Read the model definition and answer for the solid it produces. Units are mm, in the model's axes. A direction names the side the tool comes from. Give positions to 0.01 mm unless a question says otherwise; leave off trailing zeros. Order: outer loops, then holes, each group sorted by start corner. A loop starts at its lowest first (then second) coordinate and runs counter-clockwise, first axis right, second up. Notation, with made-up numbers: (-25.75, 30.25) - (18.25, 30.25) arc R3 ccw to (18.25, 34.25) - close; hole circle Ø9 at (55, 23). An arc over 180 degrees is marked (long way). Write item = value, one per line.
```python
from build123d import *

# Parameters (mm, degrees)
F0_W     = 40
F0_H     = 20
F0_R     = 10
F1_DEPTH = 30
F2_DEPTH = 30


with BuildPart() as f1:
    # F0 (on Front) → F1 (new body)
    with BuildSketch(Plane.XZ):
        with BuildLine():
            ThreePointArc((-20.300006, -30.491507), (-17.371073, -37.562575), (-10.300006, -40.491507))
            Line((-10.300006, -40.491507), (89.699994, -40.491507))
            ThreePointArc((89.699994, -40.491507), (96.771062, -37.562575), (99.699994, -30.491507))
            ThreePointArc((99.699994, -30.491507), (102.628927, -23.420439), (109.699994, -20.491507))
            Line((109.699994, -20.491507), (119.699994, -20.491507))
            ThreePointArc((119.699994, -20.491507), (126.771062, -17.562575), (129.699994, -10.491507))
            Line((129.699994, -10.491507), (129.699994, 69.508493))
            ThreePointArc((129.699994, 69.508493), (126.771062, 76.579561), (119.699994, 79.508493))
            Line((119.699994, 79.508493), (109.699994, 79.508493))
            ThreePointArc((109.699994, 79.508493), (102.628927, 82.437425), (99.699994, 89.508493))
            ThreePointArc((99.699994, 89.508493), (96.771062, 96.579561), (89.699994, 99.508493))
            Line((89.699994, 99.508493), (-10.300006, 99.508493))
            ThreePointArc((-10.300006, 99.508493), (-17.371073, 96.579561), (-20.300006, 89.508493))
            ThreePointArc((-20.300006, 89.508493), (-23.228938, 82.437425), (-30.300006, 79.508493))
            Line((-30.300006, 79.508493), (-60.300006, 79.508493))
            ThreePointArc((-60.300006, 79.508493), (-67.371073, 76.579561), (-70.300006, 69.508493))
            Line((-70.300006, 69.508493), (-70.300006, -10.491507))
            ThreePointArc((-70.300006, -10.491507), (-67.371073, -17.562575), (-60.300006, -20.491507))
            Line((-60.300006, -20.491507), (-30.300006, -20.491507))
            ThreePointArc((-30.300006, -20.491507), (-23.228938, -23.420439), (-20.300006, -30.491507))
        make_face()
        with BuildLine():
            Line((-60.300006, -11.514896), (-60.300006, 8.485104))
            Line((-60.300006, 8.485104), (-20.300006, 8.485104))
            Line((-20.300006, 8.485104), (-20.300006, -1.514896))
            ThreePointArc((-20.300006, -1.514896), (-23.228938, -8.585963), (-30.300006, -11.514896))
            Line((-30.300006, -11.514896), (-60.300006, -11.514896))
        make_face(mode=Mode.SUBTRACT)
        with Locations((-40.300006, 28.283684)):
            Rectangle(F0_W, F0_H, mode=Mode.SUBTRACT)
        with BuildLine():
            Line((67.096237, -20.491507), (7.096237, -20.491507))
            ThreePointArc((7.096237, -20.491507), (0.025169, -17.562575), (-2.903763, -10.491507))
            Line((-2.903763, -10.491507), (-2.903763, 29.508493))
            Line((-2.903763, 29.508493), (77.096237, 29.508493))
            Line((77.096237, 29.508493), (77.096237, -10.491507))
            ThreePointArc((77.096237, -10.491507), (74.167304, -17.562575), (67.096237, -20.491507))
        make_face(mode=Mode.SUBTRACT)
        with Locations((109.699994, 0)):
            Circle(F0_R, mode=Mode.SUBTRACT)
        with BuildLine():
            Line((-60.300006, 48.767287), (-60.300006, 68.767287))
            Line((-60.300006, 68.767287), (-30.300006, 68.767287))
            ThreePointArc((-30.300006, 68.767287), (-23.228938, 65.838355), (-20.300006, 58.767287))
            Line((-20.300006, 58.767287), (-20.300006, 48.767287))
            Line((-20.300006, 48.767287), (-60.300006, 48.767287))
        make_face(mode=Mode.SUBTRACT)
        with Locations((109.699994, 30)):
            Circle(F0_R, mode=Mode.SUBTRACT)
        with Locations((109.699994, 60)):
            Circle(F0_R, mode=Mode.SUBTRACT)
        with BuildLine():
            ThreePointArc((-2.903763, 69.508493), (0.025169, 76.579561), (7.096237, 79.508493))
            Line((7.096237, 79.508493), (67.096237, 79.508493))
            ThreePointArc((67.096237, 79.508493), (74.167304, 76.579561), (77.096237, 69.508493))
            Line((77.096237, 69.508493), (77.096237, 54.508493))
            Line((77.096237, 54.508493), (-2.903763, 54.508493))
            Line((-2.903763, 54.508493), (-2.903763, 69.508493))
        make_face(mode=Mode.SUBTRACT)
    extrude(amount=F1_DEPTH)

    # F0 (on Front) → F2 (join)
    with BuildSketch(Plane.XZ):
        with BuildLine():
            ThreePointArc((-20.300006, -30.491507), (-17.371073, -37.562575), (-10.300006, -40.491507))
            Line((-10.300006, -40.491507), (89.699994, -40.491507))
            ThreePointArc((89.699994, -40.491507), (96.771062, -37.562575), (99.699994, -30.491507))
            ThreePointArc((99.699994, -30.491507), (102.628927, -23.420439), (109.699994, -20.491507))
            Line((109.699994, -20.491507), (119.699994, -20.491507))
            ThreePointArc((119.699994, -20.491507), (126.771062, -17.562575), (129.699994, -10.491507))
            Line((129.699994, -10.491507), (129.699994, 69.508493))
            ThreePointArc((129.699994, 69.508493), (126.771062, 76.579561), (119.699994, 79.508493))
            Line((119.699994, 79.508493), (109.699994, 79.508493))
            ThreePointArc((109.699994, 79.508493), (102.628927, 82.437425), (99.699994, 89.508493))
            ThreePointArc((99.699994, 89.508493), (96.771062, 96.579561), (89.699994, 99.508493))
            Line((89.699994, 99.508493), (-10.300006, 99.508493))
            ThreePointArc((-10.300006, 99.508493), (-17.371073, 96.579561), (-20.300006, 89.508493))
            ThreePointArc((-20.300006, 89.508493), (-23.228938, 82.437425), (-30.300006, 79.508493))
            Line((-30.300006, 79.508493), (-60.300006, 79.508493))
            ThreePointArc((-60.300006, 79.508493), (-67.371073, 76.579561), (-70.300006, 69.508493))
            Line((-70.300006, 69.508493), (-70.300006, -10.491507))
            ThreePointArc((-70.300006, -10.491507), (-67.371073, -17.562575), (-60.300006, -20.491507))
            Line((-60.300006, -20.491507), (-30.300006, -20.491507))
            ThreePointArc((-30.300006, -20.491507), (-23.228938, -23.420439), (-20.300006, -30.491507))
        make_face()
        with BuildLine():
            Line((-60.300006, -11.514896), (-60.300006, 8.485104))
            Line((-60.300006, 8.485104), (-20.300006, 8.485104))
            Line((-20.300006, 8.485104), (-20.300006, -1.514896))
            ThreePointArc((-20.300006, -1.514896), (-23.228938, -8.585963), (-30.300006, -11.514896))
            Line((-30.300006, -11.514896), (-60.300006, -11.514896))
        make_face(mode=Mode.SUBTRACT)
        with Locations((-40.300006, 28.283684)):
            Rectangle(F0_W, F0_H, mode=Mode.SUBTRACT)
        with BuildLine():
            Line((67.096237, -20.491507), (7.096237, -20.491507))
            ThreePointArc((7.096237, -20.491507), (0.025169, -17.562575), (-2.903763, -10.491507))
            Line((-2.903763, -10.491507), (-2.903763, 29.508493))
            Line((-2.903763, 29.508493), (77.096237, 29.508493))
            Line((77.096237, 29.508493), (77.096237, -10.491507))
            ThreePointArc((77.096237, -10.491507), (74.167304, -17.562575), (67.096237, -20.491507))
        make_face(mode=Mode.SUBTRACT)
        with Locations((109.699994, 0)):
            Circle(F0_R, mode=Mode.SUBTRACT)
        with BuildLine():
            Line((-60.300006, 48.767287), (-60.300006, 68.767287))
            Line((-60.300006, 68.767287), (-30.300006, 68.767287))
            ThreePointArc((-30.300006, 68.767287), (-23.228938, 65.838355), (-20.300006, 58.767287))
            Line((-20.300006, 58.767287), (-20.300006, 48.767287))
            Line((-20.300006, 48.767287), (-60.300006, 48.767287))
        make_face(mode=Mode.SUBTRACT)
        with Locations((109.699994, 30)):
            Circle(F0_R, mode=Mode.SUBTRACT)
        with Locations((109.699994, 60)):
            Circle(F0_R, mode=Mode.SUBTRACT)
        with BuildLine():
            ThreePointArc((-2.903763, 69.508493), (0.025169, 76.579561), (7.096237, 79.508493))
            Line((7.096237, 79.508493), (67.096237, 79.508493))
            ThreePointArc((67.096237, 79.508493), (74.167304, 76.579561), (77.096237, 69.508493))
            Line((77.096237, 69.508493), (77.096237, 54.508493))
            Line((77.096237, 54.508493), (-2.903763, 54.508493))
            Line((-2.903763, 54.508493), (-2.903763, 69.508493))
        make_face(mode=Mode.SUBTRACT)
    extrude(amount=F2_DEPTH)


solid = f1.part
```
1. Flat-ended cylindrical pins translate along their axes: pin 1 (9 mm diameter, centred on x = -46, y = -12, fed in from -Z); pin 2 (5 mm diameter, centred on y = -4.5, z = 74.5, fed in from +X); pin 3 (16 mm diameter, centred on x = 109.7, z = 0, fed in from -Y); pin 4 (1 mm diameter, centred on x = 102, y = -3.5, fed in from +Z). Find the tip coordinate at first contact, or state that the pin passes through.
Recorded:
pin_1 = -20.49
pin_2 = 129.38
pin_3 = through
pin_4 = 83.78
2. Section D-D (y = -19.75) is taken. Count the separate pieces of the cut face and the enclosed holes in it, and give its area (3 significant figures).
Recorded:
separate_pieces = 1
enclosed_holes = 8
area = 15,500 mm^2
3. Determine the mould class of faces 3 (the face through (-46, -15, -20.492)), 4 (the face through (-40, -15, 48.767)) for opening direction X: +X half, -X half, draft (parallel to the pull), parting line (faces both ways), or undercut.
Recorded:
face_3 = draft
face_4 = undercut
4. Section C-C (x = -22.5) is taken. Determine the outline of the cut face in (y, z).
Recorded:
outline = (-30, -24.23) - (0, -24.23) - (0, -7.77) - (-30, -7.77) - close; (-30, 8.49) - (0, 8.49) - (0, 18.28) - (-30, 18.28) - close; (-30, 38.28) - (0, 38.28) - (0, 48.77) - (-30, 48.77) - close; (-30, 65.03) - (0, 65.03) - (0, 83.25) - (-30, 83.25) - close
5. For faces 1 (the face through (28, -30, 30)), 2 (the face through (38, -15, 54.508)), determine the directions among +Z, -Z, +X, -X, +Y, -Y from which every point of the face is accessible in a straight line to the end or side of a thin tool.
Recorded:
face_1 = +Z, -Z, +X, -X, -Y
face_2 = +Y, -Y
6. Straight lines are drawn through the part: L1, parallel to Z at x = -40, y = -22; L2, parallel to Z at x = 12.5, y = -1.25; L3, parallel to X at y = -20.75, z = 29. For each, find the intervals that lie inside material, in ascending order. Write a range as [from, to].
Recorded:
L1 = [-20.49, -11.51], [8.49, 18.28], [38.28, 48.77], [68.77, 79.51]
L2 = [-40.49, -20.49], [29.51, 54.51], [79.51, 99.51]
L3 = [-70.3, -60.3], [-20.3, -2.9], [77.1, 99.75], [119.65, 129.7]
7. Section A-A (x = 50) is taken. Determine the outline of the cut face in (y, z).
Recorded:
outline = (-30, -40.49) - (0, -40.49) - (0, -20.49) - (-30, -20.49) - close; (-30, 29.51) - (0, 29.51) - (0, 54.51) - (-30, 54.51) - close; (-30, 79.51) - (0, 79.51) - (0, 99.51) - (-30, 99.51) - close
8. Section B-B (z = 26.5) is taken. Determine the outline of the cut face in (x, y), and give its area (3 significant figures).
Recorded:
outline = (-70.3, -30) - (-60.3, -30) - (-60.3, 0) - (-70.3, 0) - close; (-20.3, -30) - (-2.9, -30) - (-2.9, 0) - (-20.3, 0) - close; (77.1, -30) - (100.33, -30) - (100.33, 0) - (77.1, 0) - close; (119.07, -30) - (129.7, -30) - (129.7, 0) - (119.07, 0) - close
area = 1,840 mm^2
